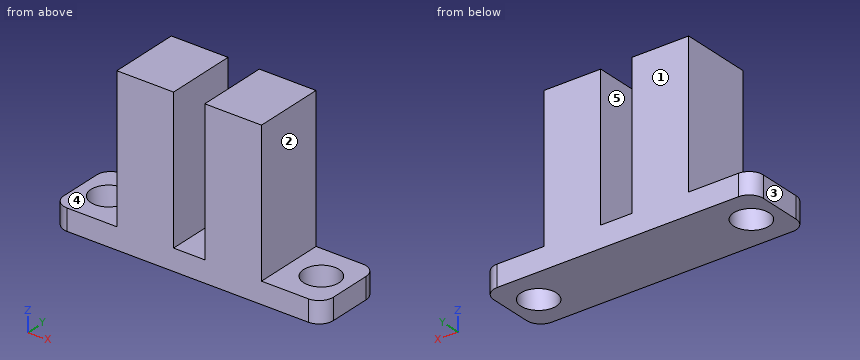
Autodesk Inventor part; units mm, degrees
ref_plane "YZ Plane" through (0, 0, 0) normal (1, 0, 0) x (0, 1, 0)
ref_plane "XZ Plane" through (0, 0, 0) normal (0, 1, 0) x (-1, 0, 0)
ref_plane "XY Plane" through (0, 0, 0) normal (0, 0, 1) x (1, 0, 0)
sketch "Náčrt1" plane through (0, 0, 0) normal (0, 0, 1) x (1, 0, 0)
  line L0 (-6.3446, 3.6092) -> (27.6554, 3.6092)
  line L1 (29.6554, 1.6092) -> (29.6554, -4.3908)
  line L2 (27.6554, -6.3908) -> (-6.3446, -6.3908)
  line L3 (-8.3446, -4.3908) -> (-8.3446, 1.6092)
  circle A0 centre (-4.3446, -1.3908) radius 2.5
  circle A1 centre (25.6554, -1.3908) radius 2.5
  arc A2 (-6.3446, 3.6092) -> (-8.3446, 1.6092) centre (-6.3446, 1.6092) ccw
  arc A3 (29.6554, 1.6092) -> (27.6554, 3.6092) centre (27.6554, 1.6092) ccw
  arc A4 (27.6554, -6.3908) -> (29.6554, -4.3908) centre (27.6554, -4.3908) ccw
  arc A5 (-8.3446, -4.3908) -> (-6.3446, -6.3908) centre (-6.3446, -4.3908) ccw
  point P0 (0, 0)
  point P1 (-8.3446, 3.6092)
  point P2 (29.6554, 3.6092)
  point P3 (-8.3446, -6.3908)
  dimension "d0" = 38
  dimension "d1" = 10
  dimension "d2" = 5
  dimension "d3" = 5
  dimension "d4" = 5
  dimension "d5" = 5
  dimension "d6" = 4
  dimension "d7" = 4
  dimension "d8" = 2
extrude "Vysunutí1" add sketch "Náčrt1" along normal blind 3
sketch "Náčrt2" plane through (0, 0, 3) normal (0, 0, 1) x (1, 0, 0)
  line L0 (0.6554, 3.6092) -> (8.6554, 3.6092)
  line L1 (8.6554, 3.6092) -> (8.6554, -6.3908)
  line L2 (8.6554, -6.3908) -> (0.6554, -6.3908)
  line L3 (0.6554, -6.3908) -> (0.6554, 3.6092)
  line L4 (13.0554, 3.6092) -> (21.0554, 3.6092)
  line L5 (21.0554, 3.6092) -> (21.0554, -6.3908)
  line L6 (21.0554, -6.3908) -> (13.0554, -6.3908)
  line L7 (13.0554, -6.3908) -> (13.0554, 3.6092)
  line L8 (-8.3446, 1.6092) -> (-8.3446, -4.3908)
  line L9 (-6.3446, -6.3908) -> (27.6554, -6.3908)
  line L10 (27.6554, 3.6092) -> (-6.3446, 3.6092)
  point P0 (0, 0)
  point P1 (4.6554, -6.3908)
  dimension "d11" = 4.4
  dimension "d12" = 8
  dimension "d13" = 8
  dimension "d14" = 9
  dimension "d15" = 10
  dimension "d16" = 0
  dimension "d21" = 0
extrude "Vysunutí2" add sketch "Náčrt2" along normal blind 20 contours L0 L1 L2 L3 | L4 L5 L6 L7
properties part number "uchytka"
Here's how the part is built. I have some questions about the finished solid (model axes, mm). Face numbers are marked on the shaded views. A direction names the side the tool comes from. Coordinates: 2 decimals unless noted, no trailing zeros. Order: outer loops, then holes, each group sorted by start corner. A loop starts at its lowest first (then second) coordinate and runs counter-clockwise, first axis right, second up. Notation, with made-up numbers: (-29.75, -12) - (-7.75, -12) arc R30 ccw to (-7.75, 21) - close; hole circle Ø7 at (32, 61). An arc over 180 degrees is marked (long way). One line per question, with ' | ' between items.
(1) Will these pins go through, and if not, where does the flat tip stop? pin 1 (1.5 mm diameter, centred on y = -0.5, z = 7.5, fed in from -X); pin 2 (3 mm diameter, centred on y = -2, z = 8.5, fed in from +X); pin 3 (3 mm diameter, centred on y = 1, z = 4, fed in from -X); pin 4 (2.5 mm diameter, centred on x = -2.5, y = 0, fed in from +Z).
Report:
pin 1: stops at x = 0.66 | pin 2: stops at x = 21.06 | pin 3: stops at x = -8.34 | pin 4: stops at z = 3
(2) Suppose I cut it at A-A on z = 9. List the corners of the cut face in (x, y) for me.
Report:
outline: (0.66, -6.39) - (8.66, -6.39) - (8.66, 3.61) - (0.66, 3.61) - close; (13.06, -6.39) - (21.06, -6.39) - (21.06, 3.61) - (13.06, 3.61) - close
(3) For the marked faces 1, 2, 3, 4 and 5, which set-ups out of +Z, -Z, +X, -X, +Y, -Y let a thin tool reach every point of the face, with its end or its side?
Report:
face 1: +Z, -Z, +X, -X, +Y | face 2: +Z, +X, +Y, -Y | face 3: +Z, -Z, -X, +Y, -Y | face 4: +Z, -X, +Y, -Y | face 5: +Z, +Y, -Y
(4) Suppose I cut it at B-B on y = 0.5. List the corners of the cut face in (x, z) for me, and give its area (3 significant figures).
Report:
outline: (-8.34, 0) - (-5.98, 0) - (-5.98, 3) - (-8.34, 3) - close; (-2.71, 0) - (24.02, 0) - (24.02, 3) - (21.06, 3) - (21.06, 23) - (13.06, 23) - (13.06, 3) - (8.66, 3) - (8.66, 23) - (0.66, 23) - (0.66, 3) - (-2.71, 3) - close; (27.29, 0) - (29.66, 0) - (29.66, 3) - (27.29, 3) - close | area: 414 mm2
(5) If I drill on L1, parallel to X at y = 1.75, z = 7.5; L2, parallel to Z at x = 22, y = 1.75, over which ranges is the centre line in solid material (lowest first)?
Report:
L1: x = 0.66 to 8.66, 13.06 to 21.06 | L2: z = 0 to 3
(6) Suppose I cut it at D-D on z = 2. List the corners of the cut face in (x, y) for me.
Report:
outline: (-8.34, -4.39) arc R2 ccw to (-6.34, -6.39) - (27.66, -6.39) arc R2 ccw to (29.66, -4.39) - (29.66, 1.61) arc R2 ccw to (27.66, 3.61) - (-6.34, 3.61) arc R2 ccw to (-8.34, 1.61) - close; hole circle Ø5 at (-4.34, -1.39); hole circle Ø5 at (25.66, -1.39)
(7) Suppose I cut it at C-C on x = 27. List the corners of the cut face in (y, z) for me.
Report:
outline: (-6.39, 0) - (-3.5, 0) - (-3.5, 3) - (-6.39, 3) - close; (0.72, 0) - (3.61, 0) - (3.61, 3) - (0.72, 3) - close
